```python
from build123d import *

# Parameters (mm, degrees)
SKETCH_1_R          = 6.5
EXTRUDE_1_DEPTH     = 7
EXTRUDE_2_DEPTH     = 6
SKETCH_4_R          = 6.5
EXTRUDE_3_DEPTH     = 1
SKETCH_5_R          = 2.5
CUT_EXTRUDE_1_DEPTH = 17.748134224


with BuildPart() as part:
    # 草图1 → 凸台-拉伸1 (new body)
    with BuildSketch(Plane.XY):
        Circle(SKETCH_1_R)
    extrude(amount=EXTRUDE_1_DEPTH)

    # 草图2 → 凸台-拉伸2 (add)
    with BuildSketch(Plane.XY.offset(7)):
        with BuildLine():
            ThreePointArc((-0.599999991, 4.683458109), (-0.655607945, 4.803813062), (-0.783301597, 4.839476633))
            ThreePointArc((-0.783301597, 4.839476633), (-0.95642213, 4.808258747), (-1.128311215, 4.770849953))
            ThreePointArc((-1.128311215, 4.770849953), (-1.232636909, 4.689034864), (-1.237954113, 4.556561144))
            ThreePointArc((-1.237954113, 4.556561144), (-1.562671768, 3.772623377), (-2.346609536, 4.097341032))
            ThreePointArc((-2.346609536, 4.097341032), (-2.444042432, 4.187254267), (-2.575663842, 4.171336866))
            ThreePointArc((-2.575663842, 4.171336866), (-2.723659792, 4.07624494), (-2.868148874, 3.975904616))
            ThreePointArc((-2.868148874, 3.975904616), (-2.933223968, 3.860393615), (-2.887440926, 3.73596905))
            ThreePointArc((-2.887440926, 3.73596905), (-2.887440926, 2.887440926), (-3.73596905, 2.887440926))
            ThreePointArc((-3.73596905, 2.887440926), (-3.860393615, 2.933223968), (-3.975904616, 2.868148874))
            ThreePointArc((-3.975904616, 2.868148874), (-4.07624494, 2.723659792), (-4.171336866, 2.575663842))
            ThreePointArc((-4.171336866, 2.575663842), (-4.187254267, 2.444042432), (-4.097341032, 2.346609535))
            ThreePointArc((-4.097341032, 2.346609535), (-3.772623377, 1.562671768), (-4.556561144, 1.237954113))
            ThreePointArc((-4.556561144, 1.237954113), (-4.689034864, 1.232636909), (-4.770849953, 1.128311215))
            ThreePointArc((-4.770849953, 1.128311215), (-4.808258747, 0.95642213), (-4.839476633, 0.783301597))
            ThreePointArc((-4.839476633, 0.783301597), (-4.803813062, 0.655607945), (-4.683458109, 0.599999991))
            ThreePointArc((-4.683458109, 0.599999991), (-4.083458118, 0), (-4.683458109, -0.599999991))
            ThreePointArc((-4.683458109, -0.599999991), (-4.803813062, -0.655607945), (-4.839476633, -0.783301597))
            ThreePointArc((-4.839476633, -0.783301597), (-4.808258747, -0.95642213), (-4.770849953, -1.128311215))
            ThreePointArc((-4.770849953, -1.128311215), (-4.689034864, -1.232636909), (-4.556561144, -1.237954113))
            ThreePointArc((-4.556561144, -1.237954113), (-3.772623377, -1.562671768), (-4.097341032, -2.346609536))
            ThreePointArc((-4.097341032, -2.346609536), (-4.187254267, -2.444042432), (-4.171336866, -2.575663842))
            ThreePointArc((-4.171336866, -2.575663842), (-4.07624494, -2.723659792), (-3.975904616, -2.868148874))
            ThreePointArc((-3.975904616, -2.868148874), (-3.860393615, -2.933223968), (-3.73596905, -2.887440926))
            ThreePointArc((-3.73596905, -2.887440926), (-2.887440926, -2.887440926), (-2.887440926, -3.73596905))
            ThreePointArc((-2.887440926, -3.73596905), (-2.933223968, -3.860393615), (-2.868148874, -3.975904616))
            ThreePointArc((-2.868148874, -3.975904616), (-2.723659792, -4.07624494), (-2.575663842, -4.171336866))
            ThreePointArc((-2.575663842, -4.171336866), (-2.444042432, -4.187254267), (-2.346609535, -4.097341032))
            ThreePointArc((-2.346609535, -4.097341032), (-1.562671768, -3.772623377), (-1.237954113, -4.556561144))
            ThreePointArc((-1.237954113, -4.556561144), (-1.232636909, -4.689034864), (-1.128311215, -4.770849953))
            ThreePointArc((-1.128311215, -4.770849953), (-0.95642213, -4.808258747), (-0.783301597, -4.839476633))
            ThreePointArc((-0.783301597, -4.839476633), (-0.655607945, -4.803813062), (-0.599999991, -4.683458109))
            ThreePointArc((-0.599999991, -4.683458109), (0, -4.083458118), (0.599999991, -4.683458109))
            ThreePointArc((0.599999991, -4.683458109), (0.655607945, -4.803813062), (0.783301597, -4.839476633))
            ThreePointArc((0.783301597, -4.839476633), (0.95642213, -4.808258747), (1.128311215, -4.770849953))
            ThreePointArc((1.128311215, -4.770849953), (1.232636909, -4.689034864), (1.237954113, -4.556561144))
            ThreePointArc((1.237954113, -4.556561144), (1.562671768, -3.772623377), (2.346609536, -4.097341032))
            ThreePointArc((2.346609536, -4.097341032), (2.444042432, -4.187254267), (2.575663842, -4.171336866))
            ThreePointArc((2.575663842, -4.171336866), (2.723659792, -4.07624494), (2.868148874, -3.975904616))
            ThreePointArc((2.868148874, -3.975904616), (2.933223968, -3.860393615), (2.887440926, -3.73596905))
            ThreePointArc((2.887440926, -3.73596905), (2.887440926, -2.887440926), (3.73596905, -2.887440926))
            ThreePointArc((3.73596905, -2.887440926), (3.860393615, -2.933223968), (3.975904616, -2.868148874))
            ThreePointArc((3.975904616, -2.868148874), (4.07624494, -2.723659792), (4.171336866, -2.575663842))
            ThreePointArc((4.171336866, -2.575663842), (4.187254267, -2.444042432), (4.097341032, -2.346609535))
            ThreePointArc((4.097341032, -2.346609535), (3.772623377, -1.562671768), (4.556561144, -1.237954113))
            ThreePointArc((4.556561144, -1.237954113), (4.689034864, -1.232636909), (4.770849953, -1.128311215))
            ThreePointArc((4.770849953, -1.128311215), (4.808258747, -0.95642213), (4.839476633, -0.783301597))
            ThreePointArc((4.839476633, -0.783301597), (4.803813062, -0.655607945), (4.683458109, -0.599999991))
            ThreePointArc((4.683458109, -0.599999991), (4.083458118, 0), (4.683458109, 0.599999991))
            ThreePointArc((4.683458109, 0.599999991), (4.803813062, 0.655607945), (4.839476633, 0.783301597))
            ThreePointArc((4.839476633, 0.783301597), (4.808258747, 0.95642213), (4.770849953, 1.128311215))
            ThreePointArc((4.770849953, 1.128311215), (4.689034864, 1.232636909), (4.556561144, 1.237954113))
            ThreePointArc((4.556561144, 1.237954113), (3.772623377, 1.562671768), (4.097341032, 2.346609536))
            ThreePointArc((4.097341032, 2.346609536), (4.187254267, 2.444042432), (4.171336866, 2.575663842))
            ThreePointArc((4.171336866, 2.575663842), (4.07624494, 2.723659792), (3.975904616, 2.868148874))
            ThreePointArc((3.975904616, 2.868148874), (3.860393615, 2.933223968), (3.73596905, 2.887440926))
            ThreePointArc((3.73596905, 2.887440926), (2.887440926, 2.887440926), (2.887440926, 3.73596905))
            ThreePointArc((2.887440926, 3.73596905), (2.933223968, 3.860393615), (2.868148874, 3.975904616))
            ThreePointArc((2.868148874, 3.975904616), (2.723659792, 4.07624494), (2.575663842, 4.171336866))
            ThreePointArc((2.575663842, 4.171336866), (2.444042432, 4.187254267), (2.346609535, 4.097341032))
            ThreePointArc((2.346609535, 4.097341032), (1.562671768, 3.772623377), (1.237954113, 4.556561144))
            ThreePointArc((1.237954113, 4.556561144), (1.232636909, 4.689034864), (1.128311215, 4.770849953))
            ThreePointArc((1.128311215, 4.770849953), (0.95642213, 4.808258747), (0.783301597, 4.839476633))
            ThreePointArc((0.783301597, 4.839476633), (0.655607945, 4.803813062), (0.599999991, 4.683458109))
            ThreePointArc((0.599999991, 4.683458109), (0, 4.083458118), (-0.599999991, 4.683458109))
        make_face()
    extrude(amount=EXTRUDE_2_DEPTH)

    # 草图4 → 凸台-拉伸3 (add)
    with BuildSketch(Plane.XY.offset(13)):
        Circle(SKETCH_4_R)
    extrude(amount=EXTRUDE_3_DEPTH)

    # 草图5 → 切除-拉伸1 (cut, through all)
    with BuildSketch(Plane(origin=(0, 0, 0), x_dir=(-1, 0, 0), z_dir=(0, 0, -1))):
        Circle(SKETCH_5_R)
    extrude(amount=-CUT_EXTRUDE_1_DEPTH, mode=Mode.SUBTRACT)


solid = part.part
```
Verification items for the finished model (mm, model axes). A direction names the side the tool comes from. Give positions to 0.01 mm unless a question says otherwise; leave off trailing zeros. Order: outer loops, then holes, each group sorted by start corner. A loop starts at its lowest first (then second) coordinate and runs counter-clockwise, first axis right, second up. Notation, with made-up numbers: M 89,22 L 126,22 A12 cw 126,30 Z; hole C -18,-38.5 d9. An arc over 180 degrees is marked long. Return JSON: item names as keys, results as strings. Group by question number.
1) Mould release check, pull along X, two halves, no side actions. Record for faces 4 (the face through (1.57, 3.77, 9.96)), 5 (the face through (3, 0, 0)), 6 (the face through (-5.158, -3.955, 13.493)): pulls with the +X half, pulls with the -X half, needs draft (parallel to the pull), parting line crosses it, or undercut.
2) Section check A-A on x = 0. Record the cut outline in (y, z).
3) Section check C-C on z = 6.5. Record the cut outline in (x, y), and give its area (3 significant figures).
4) Go/stop test with flat-tipped pins: pin 1 Ø4 at (y, z) = (2.5, 12) entering from +X; pin 2 Ø1 at (y, z) = (-4.5, 6) entering from -X. Record where each tip stops, or that it passes through.
5) Section check D-D on y = 3.25. Record the cut outline in (x, z).
6) Access from +Z, -Z, +X, -X, +Y, -Y to the whole of each face (thin tool, end or side, straight path). Record for faces 1 (the face through (4.084, -0.013, 9.958)), 2 (the face through (-1.55, 3.78, 9.96)), 3 (the face through (-4.084, 0.013, 9.958)).
7) Scan lines: line 1 (Z direction, x = 3, y = -5.25); line 2 (Y direction, x = 0, z = 10.5); line 3 (Y direction, x = -4, z = 11.75). Record each from-to range of solid material in increasing order.
Answer block:
{
 "1": {"face 4": "undercut", "face 5": "needs draft", "face 6": "parting line crosses it"},
 "2": {"outline": "M -6.5,0 L -2.5,0 L -2.5,14 L -6.5,14 L -6.5,13 L -4.08,13 L -4.08,7 L -6.5,7 Z; M 2.5,0 L 6.5,0 L 6.5,7 L 4.08,7 L 4.08,13 L 6.5,13 L 6.5,14 L 2.5,14 Z"},
 "3": {"outline": "C 0,0 d13; hole C 0,0 d5", "area": "113 mm^2"},
 "4": {"pin 1": "stops at x = 6.45", "pin 2": "stops at x = -5.12"},
 "5": {"outline": "M -5.63,0 L 5.63,0 L 5.63,7 L 2.71,7 L 2.71,13 L 5.63,13 L 5.63,14 L -5.63,14 L -5.63,13 L -2.71,13 L -2.71,7 L -5.63,7 Z"},
 "6": {"face 1": "+X", "face 2": "none", "face 3": "-X"},
 "7": {"line 1": "z = 0 to 7, 13 to 14", "line 2": "y = -4.08 to -2.5, 2.5 to 4.08", "line 3": "y = -2.83 to -2.3, -1.29 to 1.29, 2.3 to 2.83"}
}
